Work out the finished part from the listing and answer in its coordinate system (mm). A direction names the side the tool comes from. Coordinates: 2 decimals unless noted, no trailing zeros. Order: outer loops, then holes, each group sorted by start corner. A loop starts at its lowest first (then second) coordinate and runs counter-clockwise, first axis right, second up. Notation, with made-up numbers: M 41,44 L 51,44 A32 cw 51,78 Z; hole C 27.5,6 d7. An arc over 180 degrees is marked long. Write item = value, one per line. Start each with the question number.
Q1. Straight lines are drawn through the part: line 1 along X through (y, z) = (15.5, 4.75) (3 decimals); line 2 along Y through (x, z) = (-11, 1.5) (3 decimals); line 3 along Y through (x, z) = (-50, -3.5). For each, find the intervals that lie inside material, in ascending order.
Q2. Find section D-D on y = 34. Give the number of separate pieces and of enclosed holes in the cut face, and give its area (3 significant figures).
Q3. Find section B-B on x = -13. Give the vertices of the cut face in (y, z) (3 decimals), and give its area (4 significant figures).
Q4. Each of these flat-tipped pins is pushed along its axis until it touches: P1, Ø10, axis at x = 6, y = 18, coming from the -Z side; P2, Ø6.5, axis at y = 42.5, z = -0.5, coming from the -X side; P3, Ø1.2, axis at x = -60, y = -1.5, coming from the -Z side. Where does it stop, or does it pass through?
Q5. Determine the mould class of faces 1 (the cylindrical face through (-62.439, 43.296, 2.395)), 2 (the flat face through (-10, 35.575, 2)), 3 (the conical face through (34.351, -4.425, 11.208)) for opening direction Y: released by +Y, released by -Y, zero draft, split by the parting line, or undercut.
Q6. A tool of negligible diameter and unlimited length cuts with its end or side. For faces 4 (the flat face through (0, 19, 8)), 5 (the flat face through (-14, -6, 11)), 6 (the flat face through (0, 34, -2)), 7 (the flat face through (-35.575, 9, 2)), from which of +Z, -Z, +X, -X, +Y, -Y can it reach the whole face along a straight path? Write none if from no direction.
Q7. Find section C-C on z = 7.75. Give the vertices of the cut face in (x, y).
Q8. Find section A-A on y = 22.5. Give the vertices of the cut face in (x, z) (3 decimals).
```python
from build123d import *

# Parameters (mm, degrees)
SKETCH011_W       = 57.15
SKETCH011_H       = 38.1
SKETCH011_W_2     = 14
SKETCH011_H_2     = 14
PAD007_DEPTH      = 5
SKETCH012_W       = 101.15
SKETCH012_H       = 52.1
SKETCH012_W_2     = 57.15
SKETCH012_H_2     = 38.1
PAD008_DEPTH      = 12
PAD008_DEPTH_BACK = 5
FILLET001_R       = 6
POCKET005_DEPTH   = 5
SKETCH014_W       = 26
SKETCH014_H       = 35.1
POCKET006_DEPTH   = 5
SKETCH015_W       = 12
SKETCH015_H       = 7
POCKET007_DEPTH   = 7.001
FILLET002_R       = 1
CHAMFER001_SIZE   = 2
SKETCH018_R       = 2
POCKET008_DEPTH   = 6


with BuildPart() as part:
    # Sketch011 → Pad007 (new body)
    with BuildSketch(Plane.XY):
        with Locations((-28.575, 19.05)):
            Rectangle(SKETCH011_W, SKETCH011_H)
        with Locations((-47.625, 28.575)):
            Rectangle(SKETCH011_W_2, SKETCH011_H_2, mode=Mode.SUBTRACT)
        with Locations((-28.575, 28.575)):
            Rectangle(SKETCH011_W_2, SKETCH011_H_2, mode=Mode.SUBTRACT)
        with Locations((-9.525, 28.575)):
            Rectangle(SKETCH011_W_2, SKETCH011_H_2, mode=Mode.SUBTRACT)
        with Locations((-47.625, 9.525)):
            Rectangle(SKETCH011_W_2, SKETCH011_H_2, mode=Mode.SUBTRACT)
        with Locations((-28.575, 9.525)):
            Rectangle(SKETCH011_W_2, SKETCH011_H_2, mode=Mode.SUBTRACT)
        with Locations((-9.525, 9.525)):
            Rectangle(SKETCH011_W_2, SKETCH011_H_2, mode=Mode.SUBTRACT)
    extrude(amount=PAD007_DEPTH)

    # Sketch012 → Pad008 (join, two sides)
    with BuildSketch(Plane.XY) as pad008_sk:
        with Locations((-13.575, 19.05)):
            Rectangle(SKETCH012_W, SKETCH012_H)
        with Locations((-28.575, 19.05)):
            Rectangle(SKETCH012_W_2, SKETCH012_H_2, mode=Mode.SUBTRACT)
    extrude(amount=PAD008_DEPTH)
    extrude(pad008_sk.sketch, amount=-PAD008_DEPTH_BACK)

    # Fillet001
    fillet001_edges = [part.edges().sort_by_distance(p)[0] for p in [
        (37, -7, 3.5),
        (37, 45.1, 3.5),
        (-64.15, -7, 3.5),
        (-64.15, 45.1, 3.5),
    ]]
    fillet(fillet001_edges, radius=FILLET001_R)

    # Sketch013 (on Face2 of Fillet001) → Pocket005 (cut)
    with BuildSketch(Plane(origin=(0, 0, -5), x_dir=(1, 0, 0), z_dir=(0, 0, -1))):
        Polygon((5, -8), (-2.525, -8), (-2.525, -30.1), (5, -30.1), (5, -38.1), (31, -38.1), (31, -3), (5, -3), align=None)
    extrude(amount=-POCKET005_DEPTH, mode=Mode.SUBTRACT)

    # Sketch014 (on Face28 of Pocket005) → Pocket006 (cut)
    with BuildSketch(Plane(origin=(0, 0, 0), x_dir=(1, 0, 0), z_dir=(0, 0, -1))):
        with Locations((18, -20.55)):
            Rectangle(SKETCH014_W, SKETCH014_H)
    extrude(amount=-POCKET006_DEPTH, mode=Mode.SUBTRACT)

    # Sketch015 (on Face16 of Pocket006) → Pocket007 (cut, through all)
    with BuildSketch(Plane.XZ.offset(-38.1)):
        with Locations((18.5, -1.5)):
            Rectangle(SKETCH015_W, SKETCH015_H)
    extrude(amount=-POCKET007_DEPTH, mode=Mode.SUBTRACT)

    # Fillet002
    fillet002_edges = [part.edges().sort_by_distance(p)[0] for p in [
        (24.5, 41.6, 2),
        (12.5, 41.6, 2),
    ]]
    fillet(fillet002_edges, radius=FILLET002_R)

    # Chamfer001
    chamfer001_edges = [part.edges().sort_by_distance(p)[0] for p in [
        (-13.575, -7, 12),
    ]]
    chamfer(chamfer001_edges, length=CHAMFER001_SIZE)

    # Sketch018 (on Face4 of Chamfer001) → Pocket008 (cut)
    with BuildSketch(Plane(origin=(0, 0, -5), x_dir=(1, 0, 0), z_dir=(0, 0, -1))):
        with Locations((-59.564214, 2.414214)):
            Circle(SKETCH018_R)
        with Locations((32.414214, 2.414214)):
            Circle(SKETCH018_R)
        with Locations((32.414214, -40.514214)):
            Circle(SKETCH018_R)
        with Locations((-59.564214, -40.514214)):
            Circle(SKETCH018_R)
    extrude(amount=-POCKET008_DEPTH, mode=Mode.SUBTRACT)


solid = part.part
```
Findings below:
q1.line_1 = -64.15 to -54.625, -40.625 to -35.575, -21.575 to -16.525, -2.525 to 5, 31 to 37
q1.line_2 = -7 to 2.525, 16.525 to 21.575, 35.575 to 45.1
q1.line_3 = -7 to 0, 38.1 to 45.1
q2.separate_pieces = 4
q2.enclosed_holes = 0
q2.area = 560 mm^2
q3.outline = M -7,-5 L 0,-5 L 0,0 L 2.525,0 L 2.525,5 L 0,5 L 0,12 L -5,12 L -7,10 Z; M 16.525,0 L 21.575,0 L 21.575,5 L 16.525,5 Z; M 35.575,0 L 38.1,0 L 38.1,-5 L 45.1,-5 L 45.1,10 L 43.1,12 L 38.1,12 L 38.1,5 L 35.575,5 Z
q3.area = 284.5 mm^2
q4.P1 = 0
q4.P2 = -64.15
q4.P3 = 1
q5.face_1 = released by +Y
q5.face_2 = undercut
q5.face_3 = released by -Y
q6.face_4 = +Z
q6.face_5 = +Z, +X, -X, -Y
q6.face_6 = -Z
q6.face_7 = +Z, -Z
q7.outline = M -64.15,-1 A6 ccw -58.15,-7 L 31,-7 A6 ccw 37,-1 L 37,39.1 A6 ccw 31,45.1 L -58.15,45.1 A6 ccw -64.15,39.1 Z; hole M -57.15,0 L 0,0 L 0,38.1 L -57.15,38.1 Z
q8.outline = M -64.15,-5 L -57.15,-5 L -57.15,0 L -54.625,0 L -54.625,5 L -57.15,5 L -57.15,12 L -62.15,12 L -64.15,10 Z; M -40.625,0 L -35.575,0 L -35.575,5 L -40.625,5 Z; M -21.575,0 L -16.525,0 L -16.525,5 L -21.575,5 Z; M -2.525,0 L 5,0 L 5,5 L 31,5 L 31,-5 L 37,-5 L 37,10 L 35,12 L 0,12 L 0,5 L -2.525,5 Z
